```python
from build123d import *

# Parameters (mm, degrees)
EXTRUSION1_DEPTH = 14
ESQUISSE2_R      = 2
EXTRUSION2_DEPTH = 14


with BuildPart() as part:
    # Esquisse1 → Extrusion1 (new body)
    with BuildSketch(Plane.XY):
        with BuildLine():
            Line((-17, 0), (-17, 13))
            Line((-17, 13), (17, 13))
            Line((17, 13), (17, 0))
            Line((17, 0), (11, 0))
            ThreePointArc((11, 0), (0, 11), (-11, 0))
            Line((-11, 0), (-17, 0))
        make_face()
    extrude(amount=EXTRUSION1_DEPTH)

    # Esquisse2 → Extrusion2 (cut, through all)
    with BuildSketch(Plane(origin=(0, 13, 0), x_dir=(1, 0, 0), z_dir=(0, 1, 0))):
        with Locations((-14, -7)):
            Circle(ESQUISSE2_R)
        with Locations((14, -7)):
            Circle(ESQUISSE2_R)
    extrude(amount=-EXTRUSION2_DEPTH, mode=Mode.SUBTRACT)


solid = part.part
```
Can you work these out from the model? Positions are in its coordinate system, mm. Coordinates: 2 decimals unless noted, no trailing zeros. Loops run counter-clockwise (first coordinate to the right, second up) from the corner with the lowest first, then second, coordinate; pieces in that order, holes last.
1) Imagine slicing it at A-A on x = -14. List the corners of the cut face in (y, z) for me.
2) Thinking about a two-plate mould opening in X: for faces 1 (the flat face through (0, 12, 14)), 2 (the flat face through (-17, 6, 7)), 3 (the cylindrical face through (0, 11, 7)), 4 (the cylindrical face through (-15.6, 6.6, 8.2)), which applies, pulls with the +X half, pulls with the -X half, needs draft (parallel to the pull), parting line crosses it, or undercut?
3) Imagine slicing it at C-C on z = 7. List the corners of the cut face in (x, y) for me.
4) I need wall thicknesses on probe 1 along X at (y, z) = (6, 7); probe 2 along Z at (x, y) = (-14, 9.5); probe 3 along X at (y, z) = (7.5, 7). Which ranges of each line are inside material? Lowest first, please.
5) Imagine slicing it at B-B on y = 7. List the corners of the cut face in (x, z) for me.
6) Imagine slicing it at D-D on z = 9.75. List the corners of the cut face in (x, y) for me, plus the area to 3 significant figures.
7) For pin 1 (2.5 mm diameter, centred on x = 14, z = 7, fed in from -Y), with a flat end and sliding along its axis, tell me the tip position at first contact or that it passes through.
Completed:
1. outline: (0, 0) - (13, 0) - (13, 5) - (0, 5) - close; (0, 9) - (13, 9) - (13, 14) - (0, 14) - close
2. face 1: needs draft
2. face 2: pulls with the -X half
2. face 3: undercut
2. face 4: undercut
3. outline: (-17, 0) - (-16, 0) - (-16, 13) - (-17, 13) - close; (-12, 0) - (-11, 0) arc R11 cw to (11, 0) - (12, 0) - (12, 13) - (-12, 13) - close; (16, 0) - (17, 0) - (17, 13) - (16, 13) - close
4. probe 1: x = -17 to -16, -12 to -9.22, 9.22 to 12, 16 to 17
4. probe 2: z = 0 to 5, 9 to 14
4. probe 3: x = -17 to -16, -12 to -8.05, 8.05 to 12, 16 to 17
5. outline: (-17, 0) - (-8.49, 0) - (-8.49, 14) - (-17, 14) - close; (8.49, 0) - (17, 0) - (17, 14) - (8.49, 14) - close; hole circle Ø4 at (-14, 7); hole circle Ø4 at (14, 7)
6. outline: (-17, 0) - (-11, 0) arc R11 cw to (11, 0) - (17, 0) - (17, 13) - (-17, 13) - close
6. area: 252 mm2
7. pin 1: passes through
